Check sheet for the modelled part. Datum: model origin and axes. Units: mm. A direction names the side the tool comes from. Round coordinates to 2 decimals unless told otherwise and drop trailing zeros. Loops run counter-clockwise (first coordinate to the right, second up) from the corner with the lowest first, then second, coordinate; pieces in that order, holes last. Notation, with made-up numbers: (-30.75, 46) - (-22.75, 46) arc R37 cw to (-22.75, 82) - close; hole circle Ø6 at (75.25, -33.75). An arc over 180 degrees is marked (long way). Put each result on its own line as item: value. Start each with the question number.
Item 1: Draft check along X on faces 3 (the flat face through (-147.616, 1, 0)), 4 (the flat face through (16.384, 1, 0)), 5 (the flat face through (-52, 2.159, 0)). Enter one of: pulls with the +X half, pulls with the -X half, needs draft (parallel to the pull), parting line crosses it, or undercut.
Item 2: Section check B-B, the plane x = -127.5. Record the cut outline in (y, z), and give its area (3 significant figures).
Item 3: Section check C-C, the plane y = 0. Record the cut outline in (x, z), and give its area (3 significant figures).
Item 4: Material ranges on line 1 along X through (y, z) = (3.7, 0); line 2 along Z through (x, y) = (-81, 2.25); line 3 along Y through (x, z) = (-138, -0.25), recorded low to high.
Item 5: Tool access check on faces 1 (the cylindrical face through (-20.23, 3.15, -1.39)), 2 (the cylindrical face through (-64.468, -1.702, -0.901)). Record the directions out of +Z, -Z, +X, -X, +Y, -Y that give a thin tool (end or side, any length) a straight path to the whole face; none if there is none.
Item 6: Section check A-A, the plane z = 0. Record the cut outline in (x, y).
Item 7: Gauge pin test, flat ends, axial feed: pin 1 Ø1 at (x, z) = (-80.5, 0.5) entering from +Y; pin 2 Ø1 at (x, z) = (-81.5, -2.5) entering from -Y. Record the tip position at first contact, or that the pin passes through.
from build123d import *

# Parameters (mm, degrees)
SKETCH1_W                = 164
SKETCH1_H                = 3
CUT_EXTRUDE3_START       = -2
CUT_EXTRUDE3_OUTLINE_R   = 1.6
CUT_EXTRUDE3_OUTLINE_R_2 = 1.65
CUT_EXTRUDE3_DEPTH       = 3


with BuildPart() as part:
    # Sketch1 → Revolve1 (revolve)
    with BuildSketch(Plane.XY):
        with Locations((-65.615874943, -0.340909091)):
            Rectangle(SKETCH1_W, SKETCH1_H)
    revolve(axis=Axis((-147.615874943, 1.159090909, 0), (1, 0, 0)))

    # Cut-Extrude3: read off the stored shape, not the designer's step
    # Cut-Extrude3 outline → Cut-Extrude3 (cut)
    with BuildSketch(Plane(origin=(16.384125057, 4.159090909, 0), x_dir=(1, 0, 0), z_dir=(0, 1, 0)).offset(CUT_EXTRUDE3_START)):
        with Locations((-126.5, 0)):
            Circle(CUT_EXTRUDE3_OUTLINE_R)
        with Locations((-37.5, 0)):
            Circle(CUT_EXTRUDE3_OUTLINE_R_2)
        with Locations((-68, 0)):
            Circle(CUT_EXTRUDE3_OUTLINE_R)
        with Locations((-96, 0)):
            Circle(CUT_EXTRUDE3_OUTLINE_R)
        with Locations((-114.7, 0)):
            Circle(CUT_EXTRUDE3_OUTLINE_R_2)
    extrude(amount=CUT_EXTRUDE3_DEPTH, mode=Mode.SUBTRACT)


solid = part.part
Check result:
1. face 3: pulls with the -X half
1. face 4: pulls with the +X half
1. face 5: undercut
2. outline: circle Ø6 at (1.16, 0)
2. area: 28.3 mm²
3. outline: (-147.62, -2.77) - (16.38, -2.77) - (16.38, 2.77) - (-147.62, 2.77) - close
3. area: 908 mm²
4. line 1: -147.62 to -111.72, -108.52 to -99.97, -96.67 to -81.22, -78.02 to -53.22, -50.02 to -22.77, -19.47 to 16.38
4. line 2: -2.79 to -0.8, 0.8 to 2.79
4. line 3: -1.83 to 4.15
5. face 1: +Y
5. face 2: +X, -X
6. outline: (-147.62, -1.84) - (16.38, -1.84) - (16.38, 4.16) - (-19.47, 4.16) - (-19.47, 2.16) - (-22.77, 2.16) - (-22.77, 4.16) - (-50.02, 4.16) - (-50.02, 2.16) - (-53.22, 2.16) - (-53.22, 4.16) - (-78.02, 4.16) - (-78.02, 2.16) - (-81.22, 2.16) - (-81.22, 4.16) - (-96.67, 4.16) - (-96.67, 2.16) - (-99.97, 2.16) - (-99.97, 4.16) - (-108.52, 4.16) - (-108.52, 2.16) - (-111.72, 2.16) - (-111.72, 4.16) - (-147.62, 4.16) - close
7. pin 1: y = 2.16
7. pin 2: y = -1.08
